The model under review builds one solid part; all positions refer to its coordinate system, in mm. A direction names the side the tool comes from. Coordinates: 2 decimals unless noted, no trailing zeros. Loops run counter-clockwise (first coordinate to the right, second up) from the corner with the lowest first, then second, coordinate; pieces in that order, holes last. Notation, with made-up numbers: (39, 39) - (50, 39) arc R34 ccw to (50, 76) - close; hole circle Ø7 at (-39, 29.5). An arc over 180 degrees is marked (long way). Answer in a Markdown table with one row per item. Add a question column.
(1) We need section D-D on z = -28. Write out the cut boundary in (x, y) (3 decimals).
(2) For P1, Ø4, axis at y = -10, z = -10, coming from the -X side; P2, Ø1.6, axis at x = 2, y = -84, coming from the +Z side; P3, Ø1.6, axis at x = 1, z = -10.5, coming from the -Y side, all flat-tipped, find the tip position at first contact; note any pin that passes through.
(3) For line 1 along Y through (x, z) = (1.1, -20); line 2 along Y through (x, z) = (1.75, -32.5); line 3 along Z through (x, y) = (1.5, -28.5), list the stretches that pass through material, from the lowest coordinate up.
(4) We need section B-B on z = -20. Write out the cut boundary in (x, y) (3 decimals).
(5) Machinability: for faces 5 (the flat face through (2, -50, -12)), 6 (the flat face through (2, -33, -26.7)), 7 (the flat face through (2, -56, -40)), which of the approach directions +Z, -Z, +X, -X, +Y, -Y give a long, thin tool a straight path to every point of the face, cutting with its end or side? Answer none if there is none.
(6) We need section C-C on x = 2.05. Write out the cut boundary in (y, z).
(7) We need section A-A on y = -103. Write out the cut boundary in (x, z) (3 decimals).
(8) Mouldability with a two-part tool opening along Y and no side actions: class faces 1 (the flat face through (2, -25, 0)), 2 (the cylindrical face through (1.57, -24.08, -21.21)), 3 (the flat face through (2, -110, -32)), 4 (the cylindrical face through (1.57, -45.97, -21.04)) as +Y half, -Y half, draft (parallel to the pull), parting line (faces both ways), or undercut.
from build123d import *

# Parameters (mm, degrees)
SKETCH1_R           = 3.3
SKETCH1_R_2         = 2.25
SKETCH1_R_3         = 2.75
BOSS_EXTRUDE1_DEPTH = 3.175


with BuildPart() as part:
    # Sketch1 → Boss-Extrude1 (new body)
    with BuildSketch(Plane(origin=(0, 0, 0), x_dir=(0, 0, -1), z_dir=(1, 0, 0))):
        Polygon((40, 0), (0, 0), (0, -50), (25, -50), (25, -110), (40, -110), (40, -50), align=None)
        with Locations((10, -10)):
            Circle(SKETCH1_R, mode=Mode.SUBTRACT)
        with Locations((20, -16.974849628)):
            Circle(SKETCH1_R_2, mode=Mode.SUBTRACT)
        with Locations((20, -25.974849628)):
            Circle(SKETCH1_R_2, mode=Mode.SUBTRACT)
        with Locations((20, -34.974849628)):
            Circle(SKETCH1_R_2, mode=Mode.SUBTRACT)
        with Locations((20, -43.974849628)):
            Circle(SKETCH1_R_2, mode=Mode.SUBTRACT)
        with Locations((32.5, -103)):
            Circle(SKETCH1_R_3, mode=Mode.SUBTRACT)
        with BuildLine():
            Line((33.3, -26.108433688), (33.3, -40.629208547))
            ThreePointArc((33.3, -40.629208547), (30, -43.929208547), (26.7, -40.629208547))
            Line((26.7, -40.629208547), (26.7, -26.108433688))
            ThreePointArc((26.7, -26.108433688), (30, -22.808433688), (33.3, -26.108433688))
        make_face(mode=Mode.SUBTRACT)
    extrude(amount=BOSS_EXTRUDE1_DEPTH)


solid = part.part
Outcome:
| question | item | result |
|---|---|---|
| 1 | outline | (0, -110) - (3.175, -110) - (3.175, -43.254) - (0, -43.254) - close; (0, -23.484) - (3.175, -23.484) - (3.175, 0) - (0, 0) - close |
| 2 | P1 | through |
| 2 | P2 | z = -25 |
| 2 | P3 | y = -50 |
| 3 | line 1 | -50 to -46.22, -41.72 to -37.22, -32.72 to -28.22, -23.72 to -19.22, -14.72 to 0 |
| 3 | line 2 | -110 to -105.75, -100.25 to -42.78, -23.95 to 0 |
| 3 | line 3 | -40 to -33.3, -26.7 to 0 |
| 4 | outline | (0, -50) - (3.175, -50) - (3.175, -46.225) - (0, -46.225) - close; (0, -41.725) - (3.175, -41.725) - (3.175, -37.225) - (0, -37.225) - close; (0, -32.725) - (3.175, -32.725) - (3.175, -28.225) - (0, -28.225) - close; (0, -23.725) - (3.175, -23.725) - (3.175, -19.225) - (0, -19.225) - close; (0, -14.725) - (3.175, -14.725) - (3.175, 0) - (0, 0) - close |
| 5 | face 5 | +Z, +X, -X, -Y |
| 5 | face 6 | +X, -X |
| 5 | face 7 | -Z, +X, -X, +Y, -Y |
| 6 | outline | (-110, -40) - (0, -40) - (0, 0) - (-50, 0) - (-50, -25) - (-110, -25) - close; hole circle Ø5.5 at (-103, -32.5); hole circle Ø4.5 at (-43.97, -20); hole (-40.63, -33.3) - (-26.11, -33.3) arc R3.3 ccw to (-26.11, -26.7) - (-40.63, -26.7) arc R3.3 ccw to start; hole circle Ø4.5 at (-34.97, -20); hole circle Ø4.5 at (-25.97, -20); hole circle Ø4.5 at (-16.97, -20); hole circle Ø6.6 at (-10, -10) |
| 7 | outline | (0, -40) - (3.175, -40) - (3.175, -35.25) - (0, -35.25) - close; (0, -29.75) - (3.175, -29.75) - (3.175, -25) - (0, -25) - close |
| 8 | face 1 | draft |
| 8 | face 2 | undercut |
| 8 | face 3 | -Y half |
| 8 | face 4 | undercut |
